Could you check a few things on this drawing? It's one solid part, dimensions in mm from its lowest x, y, z. A direction names the side the tool comes from. Round coordinates to 2 decimals unless told otherwise and drop trailing zeros. Loops run counter-clockwise (first coordinate to the right, second up) from the corner with the lowest first, then second, coordinate; pieces in that order, holes last. Notation, with made-up numbers: M 81.25,-25 L 133.25,-25 A19 cw 133.25,-10 Z; hole C 2,-28.5 d8. An arc over 180 degrees is marked long. Answer as CSV lines item,"result".
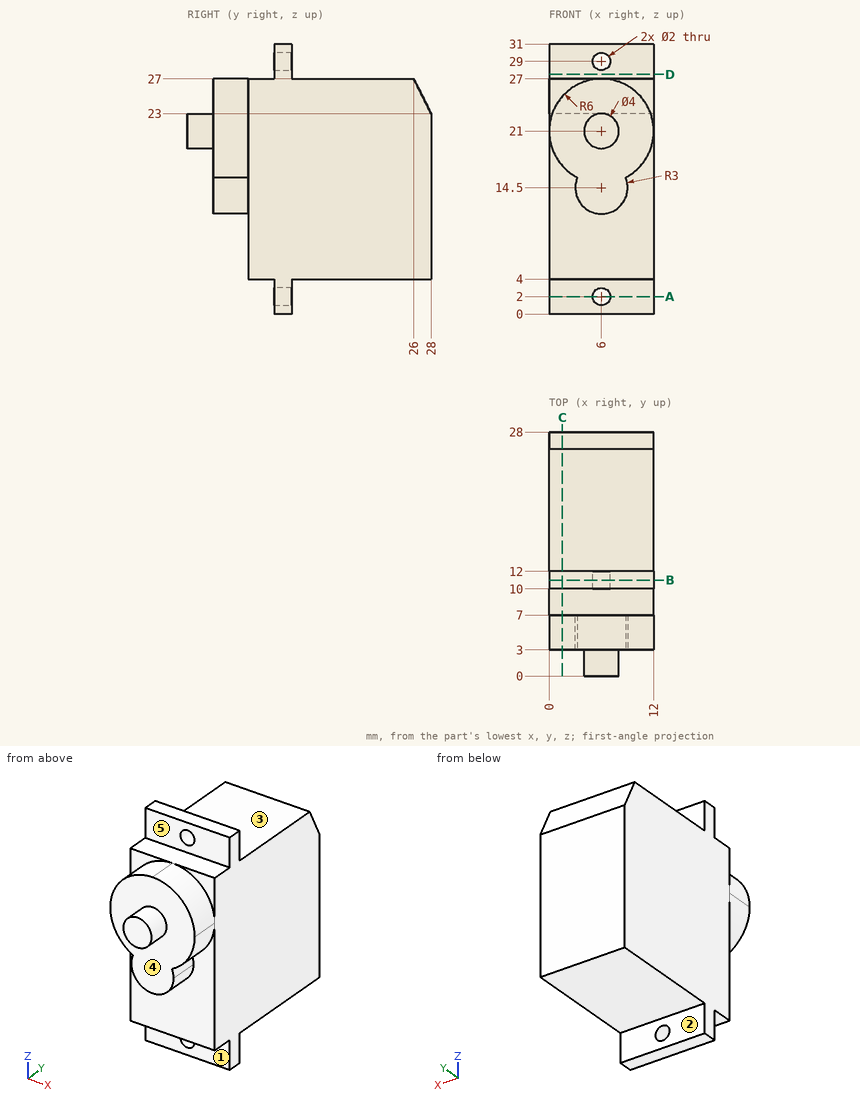
Item 1: If I drill on line 1 along X through (y, z) = (11.4, 29); line 2 along Y through (x, z) = (4.5, 25); line 3 along Y through (x, z) = (3.25, 29.5), over which ranges is the centre line in solid material (lowest first)? Write a range as from..to.
Output:
line 1,"x = 0..5, 7..12"
line 2,"y = 3..27"
line 3,"y = 10..12"
Item 2: If we section it at A-A on z = 2: Write out the boundary of the cut face in (x, y).
Output:
outline,"M 0,10 L 5,10 L 5,12 L 0,12 Z; M 7,10 L 12,10 L 12,12 L 7,12 Z"
Item 3: On a 3-axis mill with a long thin cutter (end or side, diameter ignored), from which of +Z, -Z, +X, -X, +Y, -Y can I reach the whole of each face in a straight line? I mean the marked faces 1, 2, 3, 4 and 5. Say none if no direction works.
Output:
face 1,"-Z, +X, -X, -Y"
face 2,"-Z, +X, -X, +Y"
face 3,"+Z, +X, -X, +Y"
face 4,"-Y"
face 5,"+Z, +X, -X, -Y"
Item 4: Will these pins go through, and if not, where does the flat tip stop? pin 1 (3 mm diameter, centred on x = 4.5, z = 1.5, fed in from -Y); pin 2 (2 mm diameter, centred on y = 4.5, z = 25.5, fed in from -X); pin 3 (3.5 mm diameter, centred on x = 7, z = 12.5, fed in from -Y).
Output:
pin 1,"stops at y = 10"
pin 2,"stops at x = 1.13"
pin 3,"stops at y = 3"
Item 5: If we section it at D-D on z = 27.5: Write out the boundary of the cut face in (x, y).
Output:
outline,"M 0,10 L 12,10 L 12,12 L 0,12 Z"
Item 6: If we section it at C-C on x = 1.5: Write out the boundary of the cut face in (y, z).
Output:
outline,"M 3,17.03 L 7,17.03 L 7,4 L 10,4 L 10,0 L 12,0 L 12,4 L 28,4 L 28,23 L 26,27 L 12,27 L 12,31 L 10,31 L 10,27 L 7,27 L 7,24.97 L 3,24.97 Z"
Item 7: If we section it at B-B on y = 11: Write out the boundary of the cut face in (x, z), then the cut area to 3 significant figures.
Output:
outline,"M 0,0 L 12,0 L 12,31 L 0,31 Z; hole C 6,2 d2; hole C 6,29 d2"
area,"366 mm2"
